Work out the finished part from the listing and answer in its coordinate system (mm). Give positions to 0.01 mm unless a question says otherwise; leave off trailing zeros. Write each loop counter-clockwise with the first axis right and the second up, starting at its lowest first coordinate (ties: lowest second). Pieces come first, ordered by that corner, then holes. Notation, with made-up numbers: (64, 66.5) -> (117, 66.5) arc R11 ccw to (117, 74.5) -> close; hole circle Ø4 at (43, -33). An arc over 180 degrees is marked (long way). Use a Markdown table: item, result. Add a question column.
Q1. Section B-B, the plane z = 276.5 is taken. Give the vertices of the cut face in (x, y), plus the area to 3 significant figures.
Q2. Each of these flat-tipped pins is pushed along its axis until it touches: pin 1 Ø10 at (y, z) = (-9.5, 51.5) entering from +X; pin 2 Ø3 at (x, y) = (-57, -7) entering from +Z; pin 3 Ø5 at (x, y) = (52, -16) entering from +Z. Where does it stop, or does it pass through?
Q3. Section C-C, the plane x = -68 is taken. Give the vertices of the cut face in (y, z), plus the area to 3 significant figures.
Q4. Consider line 1 (X direction, y = -11, z = 55.5); line 2 (X direction, y = -9, z = 180); line 3 (Z direction, x = -2, y = -6.75). Determine where each line is inside the solid, lowest interval first.
Q5. Section A-A, the plane y = -10.75 is taken. Give the vertices of the cut face in (x, z) (3 decimals), plus the area to 3 significant figures.
from build123d import *

# Parameters (mm, degrees)
F1_DEPTH = 18.5
F2_R     = 5
F3_R     = 5


with BuildPart() as f1:
    # F0 (on Front) → F1 (new body)
    with BuildSketch(Plane.XZ):
        with BuildLine():
            Line((-27.65, 0), (27.65, 0))
            Line((27.65, 0), (86.618847, 318.167425))
            ThreePointArc((86.618847, 318.167425), (0, 340), (-86.618847, 318.167425))
            Line((-86.618847, 318.167425), (-27.65, 0))
        make_face()
    extrude(amount=F1_DEPTH)

    # F2
    f2_edges = [f1.edges().sort_by_distance(p)[0] for p in [
        (-86.618847, -9.25, 318.167425),
    ]]
    fillet(f2_edges, radius=F2_R)

    # F3
    f3_edges = [f1.edges().sort_by_distance(p)[0] for p in [
        (86.618847, -9.25, 318.167425),
    ]]
    fillet(f3_edges, radius=F3_R)


solid = f1.part
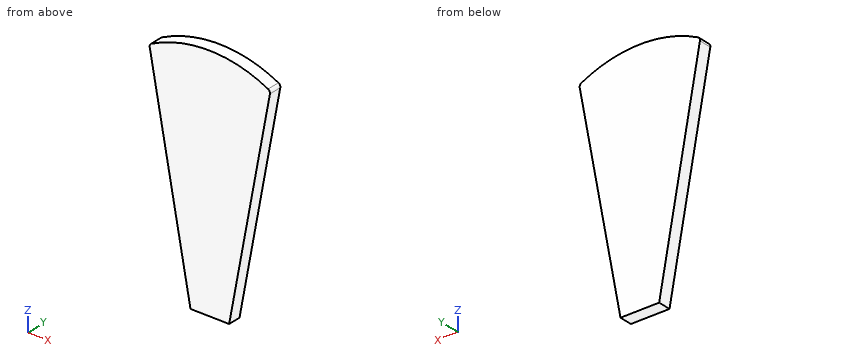
Result set:
| question | item | result |
|---|---|---|
| 1 | outline | (-78.9, -18.5) -> (78.9, -18.5) -> (78.9, 0) -> (-78.9, 0) -> close |
| 1 | area | 2,920 mm2 |
| 2 | pin 1 | stops at x = 38.12 |
| 2 | pin 2 | stops at z = 331.37 |
| 2 | pin 3 | stops at z = 333.17 |
| 3 | outline | (-18.5, 217.71) -> (0, 217.71) -> (0, 326.88) -> (-18.5, 326.88) -> close |
| 3 | area | 2,020 mm2 |
| 4 | line 1 | x = -37.94 to 37.94 |
| 4 | line 2 | x = -61.01 to 61.01 |
| 4 | line 3 | z = 0 to 339.99 |
| 5 | outline | (-85.947, 314.544) -> (-27.65, 0) -> (27.65, 0) -> (85.947, 314.544) arc R5 ccw to (83.31, 319.905) arc R182.743 ccw to (-83.31, 319.905) arc R5 ccw to start |
| 5 | area | 38,900 mm2 |
